Here's how the part is built. I have some questions about the finished solid (model axes, mm). A direction names the side the tool comes from. Coordinates: 2 decimals unless noted, no trailing zeros. Write each loop counter-clockwise with the first axis right and the second up, starting at its lowest first coordinate (ties: lowest second). Pieces come first, ordered by that corner, then holes. Notation, with made-up numbers: (22, 41.25) -> (71, 41.25) arc R25 ccw to (71, 55.25) -> close; hole circle Ø11 at (37, 49.5). An arc over 180 degrees is marked (long way). Put each result on its own line as item: value.
```python
from build123d import *

# Parameters (mm, degrees)
SKETCH1_R           = 12.7
SKETCH1_R_2         = 6.35
EXTRUDE_THIN1_DEPTH = 12.7
BOSS_EXTRUDE1_START = -12.7
BOSS_EXTRUDE1_DEPTH = 12.7
SKETCH3_R           = 19.05
BOSS_EXTRUDE2_DEPTH = 19.05
SKETCH4_R           = 12.7
CUT_EXTRUDE1_DEPTH  = 6.35


with BuildPart() as part:
    # Sketch1 → Extrude-Thin1 (new body)
    with BuildSketch(Plane(origin=(0, 0, 0), x_dir=(0, 0, -1), z_dir=(1, 0, 0))):
        Circle(SKETCH1_R)
        Circle(SKETCH1_R_2, mode=Mode.SUBTRACT)
    extrude(amount=EXTRUDE_THIN1_DEPTH)

    # Sketch2 → Boss-Extrude1 (add)
    with BuildSketch(Plane(origin=(12.7, 0, 0), x_dir=(0, 0, -1), z_dir=(1, 0, 0)).offset(BOSS_EXTRUDE1_START)):
        with BuildLine():
            Line((0, 12.7), (31.75, 12.7))
            Line((31.75, 12.7), (31.75, -12.7))
            Line((31.75, -12.7), (0, -12.7))
            ThreePointArc((0, -12.7), (12.7, 0), (0, 12.7))
        make_face()
    extrude(amount=BOSS_EXTRUDE1_DEPTH)

    # Sketch3 → Boss-Extrude2 (add)
    with BuildSketch(Plane(origin=(0, 0, -31.75), x_dir=(-1, 0, 0), z_dir=(0, 0, -1))):
        with Locations(Location((-6.35, 0, 0), (0, 0, 180))):
            Circle(SKETCH3_R)
    extrude(amount=BOSS_EXTRUDE2_DEPTH)

    # Sketch4 → Cut-Extrude1 (cut)
    with BuildSketch(Plane(origin=(0, 0, -50.8), x_dir=(-1, 0, 0), z_dir=(0, 0, -1))):
        with Locations((-6.35, 0)):
            Circle(SKETCH4_R)
    extrude(amount=-CUT_EXTRUDE1_DEPTH, mode=Mode.SUBTRACT)


solid = part.part
```
Item 1: Which directions (+Z, -Z, +X, -X, +Y, -Y) give clear straight access to the entire face, cutting with the end or side of a thin tool? Please do faces 5 (the flat face through (6, -12.7, -16)), 6 (the cylindrical face through (6.261, 0.279, 12.697)), 7 (the flat face through (12.7, 0, -15)).
Output:
face 5: +Z, +X, -X, -Y
face 6: +Z, +X, -X
face 7: +Z, +X, +Y, -Y
Item 2: If we mould it in two halves opening along Y, with no side actions, what happens to faces 1 (the cylindrical face through (-5.764, 3.815, -47.669)), 2 (the flat face through (0, 0, -15)), 3 (the flat face through (7, 0, -44.45)), 4 (the flat face through (6, 12.7, -16))? For each: released by +Y, released by -Y, zero draft, split by the parting line, or undercut.
Output:
face 1: undercut
face 2: zero draft
face 3: undercut
face 4: released by +Y
Item 3: Imagine slicing it at D-D on z = -12. Write out the boundary of the cut face in (x, y).
Output:
outline: (0, -12.7) -> (12.7, -12.7) -> (12.7, 12.7) -> (0, 12.7) -> close
Item 4: Imagine slicing it at B-B on x = 6.35. Write out the boundary of the cut face in (y, z), then the cut area to 3 significant figures.
Output:
outline: (-19.05, -50.8) -> (-12.7, -50.8) -> (-12.7, -44.45) -> (12.7, -44.45) -> (12.7, -50.8) -> (19.05, -50.8) -> (19.05, -31.75) -> (12.7, -31.75) -> (12.7, 0) arc R12.7 ccw to (-12.7, 0) -> (-12.7, -31.75) -> (-19.05, -31.75) -> close; hole circle Ø12.7 at (0, 0)
area: 1,500 mm²
Item 5: Imagine slicing it at A-A on y = 0. Write out the boundary of the cut face in (x, z).
Output:
outline: (-12.7, -50.8) -> (-6.35, -50.8) -> (-6.35, -44.45) -> (19.05, -44.45) -> (19.05, -50.8) -> (25.4, -50.8) -> (25.4, -31.75) -> (12.7, -31.75) -> (12.7, -6.35) -> (0, -6.35) -> (0, -31.75) -> (-12.7, -31.75) -> close; (0, 6.35) -> (12.7, 6.35) -> (12.7, 12.7) -> (0, 12.7) -> close
Item 6: Please list where these lines run through material, in increasing order: line 1 along Y through (x, z) = (4, 0); line 2 along Y through (x, z) = (6.35, -48.75); line 3 along Z through (x, y) = (-5.5, -11). Write a range as from..to.
Output:
line 1: y = -12.7..-6.35, 6.35..12.7
line 2: y = -19.05..-12.7, 12.7..19.05
line 3: z = -50.8..-31.75
Item 7: Imagine slicing it at C-C on z = -46. Write out the boundary of the cut face in (x, y), then the cut area to 3 significant figures.
Output:
outline: circle Ø38.1 at (6.35, 0); hole circle Ø25.4 at (6.35, 0)
area: 633 mm²
Item 8: For P1, Ø20.5, axis at y = -6, z = -8.5, coming from the -X side; P2, Ø20.5, axis at x = 10, y = -5, coming from the -Z side; P3, Ø3, axis at x = 12, z = -13.5, coming from the +Y side; P4, Ø12, axis at x = 16.5, z = -34, coming from the -Y side, each with a flat end and sliding along its axis, tell me the tip position at first contact or that it passes through.
Output:
P1: stops at x = 0
P2: stops at z = -50.8
P3: stops at y = 12.7
P4: stops at y = -18.59
